Here's how the part is built. I have some questions about the finished solid (model axes, mm). Give positions to 0.01 mm unless a question says otherwise; leave off trailing zeros. Write each loop counter-clockwise with the first axis right and the second up, starting at its lowest first coordinate (ties: lowest second). Pieces come first, ordered by that corner, then holes. Notation, with made-up numbers: (52, 85) -> (101, 85) arc R25 cw to (101, 118) -> close; hole circle Ø7 at (80.25, -7). An arc over 180 degrees is marked (long way). Use CSV: the item, a comma, the result in double quotes. Start each with the question number.
(1) Suppose I cut it at A-A on x = 0. List the corners of the cut face in (y, z) for me (3 decimals), plus the area to 3 significant figures.
(2) For pin 1 Ø3.5 at (x, z) = (0, 15.875) entering from -Y; pin 2 Ø8 at (x, z) = (4.5, -4) entering from -Y, each with a flat end and sliding along its axis, tell me the tip position at first contact or that it passes through.
(3) Suppose I cut it at B-B on z = 0. List the corners of the cut face in (x, y) for me (1 decimal).
(4) Suppose I cut it at D-D on x = 6.5. List the corners of the cut face in (y, z) for me (1 decimal), plus the area to 3 significant figures.
(5) I need wall thicknesses on L1, parallel to Z at x = 0, y = 1.65 (3 decimals); L2, parallel to X at y = 2.1, z = -17.5; L3, parallel to X at y = 0.3, z = -17. Which ranges of each line are inside material? Lowest first, please. Write a range as [from, to].
(6) Suppose I cut it at C-C on y = 1.4. Give the number of separate pieces and of enclosed holes in the cut face, plus the area to 3 significant figures.
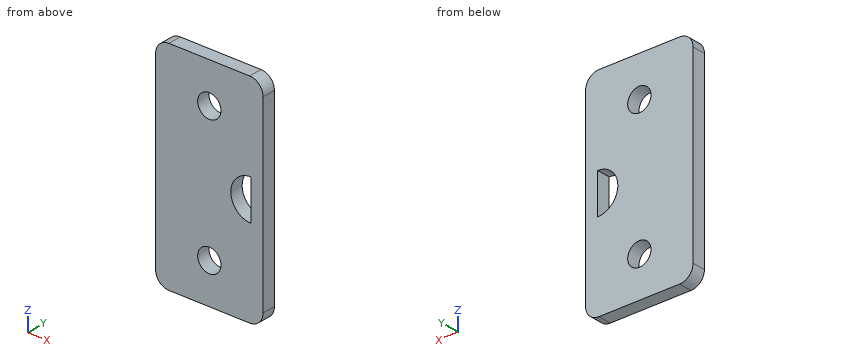
from build123d import *

# Parameters (mm, degrees)
SKETCH1_W            = 25.4
SKETCH1_H            = 50.8
BOSS_EXTRUDE1_DEPTH  = 3.175
CUT_EXTRUDE2_DEPTH   = 29.575
M5_CLEARANCE_HOLE1_D = 5.5
FILLET1_R            = 3.175


with BuildPart() as part:
    # Sketch1 → Boss-Extrude1 (new body)
    with BuildSketch(Plane(origin=(0, 0, 0), x_dir=(1, 0, 0), z_dir=(0, 1, 0))):
        Rectangle(SKETCH1_W, SKETCH1_H)
    extrude(amount=BOSS_EXTRUDE1_DEPTH)

    # Sketch8 → Cut-Extrude2 (cut, through all)
    with BuildSketch(Plane.XZ):
        with BuildLine():
            Line((9.8425, 4.7625), (9.8425, -4.7625))
            ThreePointArc((9.8425, -4.7625), (5.08, 0), (9.8425, 4.7625))
        make_face()
    extrude(amount=-CUT_EXTRUDE2_DEPTH, mode=Mode.SUBTRACT)

    # M5 Clearance Hole1 (through all)
    with Locations(Plane(origin=(0, 0, 0), x_dir=(-1, 0, 0), z_dir=(0, -1, 0))):
        with Locations((0, 15.875), (0, -15.875)):
            Hole(M5_CLEARANCE_HOLE1_D / 2)

    # Fillet1
    fillet1_edges = [part.edges().sort_by_distance(p)[0] for p in [
        (12.7, 1.5875, 25.4),
        (-12.7, 1.5875, 25.4),
        (-12.7, 1.5875, -25.4),
        (12.7, 1.5875, -25.4),
    ]]
    fillet(fillet1_edges, radius=FILLET1_R)


solid = part.part
Geometry says:
1,outline,"(0, -25.4) -> (3.175, -25.4) -> (3.175, -18.625) -> (0, -18.625) -> close; (0, -13.125) -> (3.175, -13.125) -> (3.175, 13.125) -> (0, 13.125) -> close; (0, 18.625) -> (3.175, 18.625) -> (3.175, 25.4) -> (0, 25.4) -> close"
1,area,"126 mm²"
2,pin 1,"through"
2,pin 2,"y = 0"
3,outline,"(-12.7, 0) -> (5.1, 0) -> (5.1, 3.2) -> (-12.7, 3.2) -> close; (9.8, 0) -> (12.7, 0) -> (12.7, 3.2) -> (9.8, 3.2) -> close"
4,outline,"(0, -25.4) -> (3.2, -25.4) -> (3.2, -3.4) -> (0, -3.4) -> close; (0, 3.4) -> (3.2, 3.4) -> (3.2, 25.4) -> (0, 25.4) -> close"
4,area,"140 mm²"
5,L1,"[-25.4, -18.625], [-13.125, 13.125], [18.625, 25.4]"
5,L2,"[-12.7, -2.22], [2.22, 12.7]"
5,L3,"[-12.7, -2.51], [2.51, 12.7]"
6,separate pieces,"1"
6,enclosed holes,"3"
6,area,"1,200 mm²"
